from build123d import *

# Parameters (mm, degrees)
SKETCH_1_R          = 62
SKETCH_1_R_2        = 60
EXTRUDE_1_DEPTH     = 3
EXTRUDE_START       = 6
SKETCH_2_R          = 48
EXTRUDE_2_DEPTH     = 6
FILLET_1_R          = 5
CHAMFER_1_SIZE      = 0.5
CHAMFER_2_SIZE      = 0.5
SKETCH_6_R          = 2.2
CUT_EXTRUDE_1_DEPTH = 6
SKETCH_7_W          = 65
SKETCH_7_H          = 13.477482046
EXTRUDE_3_DEPTH     = 3
SKETCH_11_R         = 1.65
CUT_EXTRUDE_2_DEPTH = 3
CHAMFER_3_SIZE      = 1
CHAMFER_4_SIZE      = 1
FILLET_2_R          = 3
CHAMFER_5_3_ANGLE   = 291.929687
SKETCH_12_R         = 4
CUT_EXTRUDE_3_DEPTH = 3


with BuildPart() as part:
    # 草图1 → 凸台-拉伸1 (new body)
    with BuildSketch(Plane.XY):
        Circle(SKETCH_1_R)
        Circle(SKETCH_1_R_2, mode=Mode.SUBTRACT)
    extrude(amount=-EXTRUDE_1_DEPTH)

    # 草图2 → 凸台-拉伸2 (add)
    with BuildSketch(Plane.XY.offset(EXTRUDE_START)):
        with BuildLine():
            Line((-32.5, 63), (32.5, 63))
            Line((32.5, 63), (32.5, 52.79914772))
            ThreePointArc((32.5, 52.79914772), (0, -62), (-32.5, 52.79914772))
            Line((-32.5, 52.79914772), (-32.5, 63))
        make_face()
        Circle(SKETCH_2_R, mode=Mode.SUBTRACT)
    extrude(amount=-EXTRUDE_2_DEPTH)

    # 圆角1
    # the kernel refuses this fillet: 5 mm, written as the material it adds along each edge
    with BuildSketch(Plane(origin=(32.5, 52.79914772, 6), x_dir=(0.8403342947446245, -0.5420685132675156, 0), z_dir=(0, 0, -1))) as fillet_1_piece_1:
        with BuildLine():
            CenterArc((2.72541822, -4.998883971), FILLET_1_R, 91.210593649, 55.964843523)
            Line((-1.476253254, -2.288541405), (0, 0))
            ThreePointArc((0, 0), (1.309890927, -0.013838756), (2.619781855, 0))
        make_face()
    extrude(amount=6)
    with BuildSketch(Plane(origin=(-32.5, 52.79914772, 6), x_dir=(-0.840334294744627, -0.5420685132675117, 0), z_dir=(0, 0, -1))) as fillet_1_piece_2:
        with BuildLine():
            CenterArc((2.72541822, 4.998883971), FILLET_1_R, 212.824562828, 55.964843523)
            Line((-1.476253254, 2.288541405), (0, 0))
            ThreePointArc((0, 0), (1.309890927, 0.013838756), (2.619781855, 0))
        make_face()
    extrude(amount=6)

    # 倒角1
    chamfer_1_edges = [part.edges().sort_by_distance(p)[0] for p in [
        (-48, 0, 0),
        (-48, 0, 6),
        (-60, 0, -3),
    ]]
    chamfer(chamfer_1_edges, length=CHAMFER_1_SIZE)

    # 倒角2
    # the kernel refuses this chamfer: 0.5 mm, written as the material it takes off along each edge
    with BuildSketch(Plane(origin=(-32.5, 55.522517954, 0), x_dir=(0, 0, 1), z_dir=(0, 1, 0)), Plane(origin=(32.5, 64.285841494, 0), x_dir=(0, 0, 1), z_dir=(0, -1, 0))) as chamfer_2_piece_1:
        Polygon((CHAMFER_2_SIZE, 0), (0, CHAMFER_2_SIZE), (0, 0), align=None)
    extrude(amount=8.76332354, mode=Mode.SUBTRACT)
    with BuildSketch(Plane(origin=(37.5, 55.522517954, 0), x_dir=(-0.15613015555825177, -0.9877364904291813, 0), z_dir=(0.9877364904291813, -0.15613015555825177, 0))) as chamfer_2_piece_2_section:
        Polygon((5, -CHAMFER_2_SIZE), (5 + CHAMFER_2_SIZE, 0), (5, 0), align=None)
    chamfer_2_piece_2 = revolve(axis=Axis((37.5, 55.522517954, 0), (0, 0, -1)), revolution_arc=81.017652556, mode=Mode.PRIVATE)
    chamfer_2_piece_2 = chamfer_2_piece_2 - Plane(origin=(0, 0, 0), x_dir=(1, 0, 0), z_dir=(0, 0, 1)) * Cylinder(62, 22, mode=Mode.PRIVATE)
    add(chamfer_2_piece_2, mode=Mode.SUBTRACT)
    with BuildSketch(Plane(origin=(-37.5, 55.522517954, 0), x_dir=(1, 0, 0), z_dir=(0, 1, 0))) as chamfer_2_piece_3_section:
        Polygon((5, -CHAMFER_2_SIZE), (5 + CHAMFER_2_SIZE, 0), (5, 0), align=None)
    chamfer_2_piece_3 = revolve(axis=Axis((-37.5, 55.522517954, 0), (0, 0, -1)), revolution_arc=81.017652556, mode=Mode.PRIVATE)
    chamfer_2_piece_3 = chamfer_2_piece_3 - Plane(origin=(0, 0, 0), x_dir=(1, 0, 0), z_dir=(0, 0, 1)) * Cylinder(62, 22, mode=Mode.PRIVATE)
    add(chamfer_2_piece_3, mode=Mode.SUBTRACT)

    # 草图6 → 切除-拉伸1 (cut)
    with BuildSketch(Plane(origin=(0, 0, 0), x_dir=(-1, 0, 0), z_dir=(0, 0, -1))):
        with Locations((-42.877900702, 31.152618372)):
            Circle(SKETCH_6_R)
        with Locations((-53, 0)):
            Circle(SKETCH_6_R)
        with Locations((-42.877900702, -31.152618371)):
            Circle(SKETCH_6_R)
        with Locations((-16.377900702, -50.405995364)):
            Circle(SKETCH_6_R)
        with Locations((16.377900702, -50.405995364)):
            Circle(SKETCH_6_R)
        with Locations((42.877900702, -31.152618371)):
            Circle(SKETCH_6_R)
        with Locations((53, 0)):
            Circle(SKETCH_6_R)
        with Locations((42.877900702, 31.152618372)):
            Circle(SKETCH_6_R)
        with Locations((16.377900702, 50.405995364)):
            Circle(SKETCH_6_R)
        with Locations((-16.377900702, 50.405995364)):
            Circle(SKETCH_6_R)
    extrude(amount=-CUT_EXTRUDE_1_DEPTH, mode=Mode.SUBTRACT)

    # 草图7 → 凸台-拉伸3 (add)
    with BuildSketch(Plane.XY.offset(6)):
        with Locations((0, 62.261258977)):
            Rectangle(SKETCH_7_W, SKETCH_7_H)
    extrude(amount=EXTRUDE_3_DEPTH)

    # 草图11 → 切除-拉伸2 (cut)
    with BuildSketch(Plane.XY.offset(9)):
        with Locations((-29.5, 66)):
            Circle(SKETCH_11_R)
        with Locations((29.5, 66)):
            Circle(SKETCH_11_R)
    extrude(amount=-CUT_EXTRUDE_2_DEPTH, mode=Mode.SUBTRACT)

    # 倒角3
    chamfer_3_edges = [part.edges().sort_by_distance(p)[0] for p in [
        (0, 63, 0),
    ]]
    chamfer(chamfer_3_edges, length=CHAMFER_3_SIZE - 0.0001)  # a hair under: the kernel refuses the full size

    # 倒角4
    chamfer_4_edges = [part.edges().sort_by_distance(p)[0] for p in [
        (0, 55.522517954, 9),
    ]]
    chamfer(chamfer_4_edges, length=CHAMFER_4_SIZE)

    # 圆角2
    fillet_2_edges = [part.edges().sort_by_distance(p)[0] for p in [
        (-32.5, 69, 7.5),
        (32.5, 69, 7.5),
    ]]
    fillet(fillet_2_edges, radius=FILLET_2_R)

    # 倒角5: read off the stored shape, not the designer's step
    # 倒角5 outline → 倒角5 (revolve, cut)
    with BuildSketch(Plane(origin=(37.5, 55.522517954, 0), x_dir=(1, 0, 0), z_dir=(0, -1, 0))):
        Polygon((4.999998721, 9), (4.999998721, 4.999998721), (9, 9), align=None)
    revolve(axis=Axis((37.5, 55.522517954, 0), (0, 0, 1)), mode=Mode.SUBTRACT)

    # Chamfer 5 2 outline → Chamfer 5 2 (revolve, cut)
    with BuildSketch(Plane(origin=(-37.5, 55.522517954, 0), x_dir=(1, 0, 0), z_dir=(0, -1, 0))):
        Polygon((4.99999762, 9), (4.99999762, 4.99999762), (9, 9), align=None)
    revolve(axis=Axis((-37.5, 55.522517954, 0), (0, 0, 1)), mode=Mode.SUBTRACT)

    # Chamfer 5 3 outline → Chamfer 5 3 (revolve, cut)
    with BuildSketch(Plane(origin=(0, 0, 0), x_dir=(-0.5597014925373135, 0.8286942978273132, 0), z_dir=(0.8286942978273132, 0.5597014925373135, 0))):
        Polygon((62, 6), (61, 6), (62, 5), align=None)
    revolve(axis=Axis((0, 0, 0), (0, 0, 1)), revolution_arc=CHAMFER_5_3_ANGLE, mode=Mode.SUBTRACT)

    # 草图12 → 切除-拉伸3 (cut)
    with BuildSketch(Plane.XY.offset(6)):
        with Locations((-16.377900702, 50.405995364)):
            Circle(SKETCH_12_R)
        with Locations((16.377900702, 50.405995364)):
            Circle(SKETCH_12_R)
        with Locations((42.877900702, 31.152618372)):
            Circle(SKETCH_12_R)
        with Locations((53, 0)):
            Circle(SKETCH_12_R)
        with Locations((42.877900702, -31.152618371)):
            Circle(SKETCH_12_R)
        with Locations((16.377900702, -50.405995364)):
            Circle(SKETCH_12_R)
        with Locations((-16.377900702, -50.405995364)):
            Circle(SKETCH_12_R)
        with Locations((-42.877900702, -31.152618371)):
            Circle(SKETCH_12_R)
        with Locations((-53, 0)):
            Circle(SKETCH_12_R)
        with Locations((-42.877900702, 31.152618372)):
            Circle(SKETCH_12_R)
    extrude(amount=-CUT_EXTRUDE_3_DEPTH, mode=Mode.SUBTRACT)


solid = part.part
Work out the finished part from the listing and answer in its coordinate system (mm). A direction names the side the tool comes from. Give positions to 0.01 mm unless a question says otherwise; leave off trailing zeros. Use a Markdown table: item, result. Add a question column.
1. Determine the mould class of faces 5 (the cylindrical face through (-17.39, -52.36, 1.48)), 6 (the cylindrical face through (-44.061, -29.298, 1.479)), 7 (the cylindrical face through (59.516, -17.375, 1.056)), 8 (the flat face through (-11.1, 61.4, 0)) for opening direction Y: released by +Y, released by -Y, zero draft, split by the parting line, or undercut.
2. For faces 1 (the flat face through (-14.7, -52.1, 3)), 2 (the flat face through (32.5, 61, 5)), 3 (the cylindrical face through (-50.802, 0.097, 1.479)), 4 (the flat face through (0, 63, 4)), determine the directions among +Z, -Z, +X, -X, +Y, -Y from which every point of the face is accessible in a straight line to the end or side of a thin tool.
3. Section A-A on y = 0 is taken. State how many separate pieces and enclosed holes the cut face has, and give its area (3 significant figures).
4. Find the intervals of material crossed by probe 1 along Y at (x, z) = (-42, 4); probe 2 along X at (y, z) = (-35, 1); probe 3 along Z at (x, y) = (-47, 34.5), in increasing order.
5. Flat-ended cylindrical pins translate along their axes: pin 1 Ø5.5 at (x, z) = (-8.5, 3) entering from +Y; pin 2 Ø9 at (x, y) = (-16, 50) entering from +Z; pin 3 Ø2.5 at (x, y) = (16.38, 50.41) entering from -Z; pin 4 Ø2.5 at (x, y) = (-54, -1.5) entering from +Z. Find the tip coordinate at first contact, or state that the pin passes through.
Results below:
| question | item | result |
|---|---|---|
| 1 | face 5 | undercut |
| 1 | face 6 | undercut |
| 1 | face 7 | split by the parting line |
| 1 | face 8 | zero draft |
| 2 | face 1 | +Z |
| 2 | face 2 | +Z, -Z, +X, +Y |
| 2 | face 3 | +Z, -Z |
| 2 | face 4 | -Z, +X, -X, +Y |
| 3 | separate pieces | 4 |
| 3 | enclosed holes | 0 |
| 3 | area | 104 mm^2 |
| 4 | probe 1 | y = -45.61 to -35.06, -27.25 to -23.24, 23.24 to 27.25, 35.06 to 45.61 |
| 4 | probe 2 | x = -51.18 to -32.85, 32.85 to 51.18 |
| 4 | probe 3 | z = 0 to 6 |
| 5 | pin 1 | stops at y = 63 |
| 5 | pin 2 | stops at z = 6 |
| 5 | pin 3 | passes through |
| 5 | pin 4 | stops at z = 3 |
